Can you work these out from the model? Positions are in its coordinate system, mm. Face numbers are marked on the shaded views. Round coordinates to 2 decimals unless told otherwise and drop trailing zeros. Write each loop counter-clockwise with the first axis right and the second up, starting at its lowest first coordinate (ties: lowest second). Pieces come first, ordered by that corner, then holes. Notation, with made-up numbers: M 64,50.5 L 93,50.5 A16 cw 93,60.5 Z; hole C -27,69.25 d11. An arc over 180 degrees is marked long. Answer as a JSON object with one key per item and string values. Group by question number.
1) Suppose I cut it at A-A, the plane y = 0. Write out the boundary of the cut face in (x, z).
2) If we mould it in two halves opening along Y, with no side actions, what happens to the marked faces 1, 2 and 3? For each: +Y half, -Y half, draft (parallel to the pull), parting line (faces both ways), or undercut.
3) Please list where these lines run through material, in increasing order: L1, parallel to Z at x = 14, y = 0; L2, parallel to Z at x = -17, y = 4.5; L3, parallel to Y at x = -6.5, z = 1. Write a range as [from, to].
4) Suppose I cut it at C-C, the plane x = -7. Write out the boundary of the cut face in (y, z).
5) I'm going to push flat-ended pins straight in: pin 1 Ø2 at (x, z) = (1.5, 4) entering from -Y; pin 2 Ø6 at (y, z) = (-1, 0) entering from -X; pin 3 Ø2 at (x, z) = (19, 2) entering from +Y; pin 4 Ø3 at (x, y) = (0, 4) entering from -Z. Where does each tip first touch, or does it pass through?
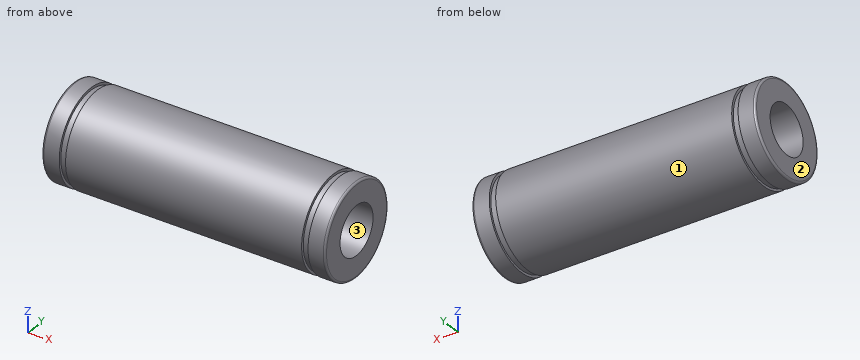
Autodesk Inventor part; units mm, degrees
ref_plane "to_housing_XY" through (0, 0, 0) normal (-1, 0, 0) x (0, 0, -1)
ref_plane "to_housing_YZ" through (0, 0, 0) normal (0, 0, -1) x (0, -1, 0)
ref_plane "to_housing_ZX" through (0, 0, 0) normal (0, -1, 0) x (-1, 0, 0)
sketch "Sketch_1" plane through (0, 0, 0) normal (0, 0, 1) x (1, 0, 0)
  line L0 (28.85, 0) -> (-28.85, 0)
  line L1 (-28.85, 0) -> (-28.85, 9.1)
  arc A0 (-28.45, 9.5) -> (-28.85, 9.1) centre (-28.45, 9.1) ccw
  line L2 (-28.45, 9.5) -> (-25.35, 9.5)
  line L3 (-25.35, 9.5) -> (-25.35, 9)
  line L4 (-25.35, 9) -> (-24.05, 9)
  line L5 (-24.05, 9) -> (-24.05, 9.5)
  line L6 (-24.05, 9.5) -> (24.05, 9.5)
  line L7 (24.05, 9.5) -> (24.05, 9)
  line L8 (24.05, 9) -> (25.35, 9)
  line L9 (25.35, 9) -> (25.35, 9.5)
  line L10 (25.35, 9.5) -> (28.45, 9.5)
  arc A1 (28.85, 9.1) -> (28.45, 9.5) centre (28.45, 9.1) ccw
  line L11 (28.85, 9.1) -> (28.85, 0)
  line L12 (28.85, 0) -> (-28.85, 0)
revolve "Revolution1" add sketch "Sketch_1" angle 360 about axis through (28.85, 0, 0) along (1, 0, 0)
sketch "Sketch2" plane through (28.85, 0, 0) normal (1, 0, 0) x (0, 0, -1)
  point P0 (0, 0)
hole "Hole1" at (28.85, 0, 0) direction (-1, 0, 0) diameter 10 depth 57.7
ref_plane "to_housing_XY" through (0, 0, 0) normal (-1, 0, 0) x (0, 0, -1)
ref_plane "to_housing_YZ" through (0, 0, 0) normal (0, 0, -1) x (0, -1, 0)
ref_plane "to_housing_ZX" through (0, 0, 0) normal (0, -1, 0) x (-1, 0, 0)
properties part number "BUSHING_REFERENCE_DATA_FOR_LHSSW10"
Results:
{
 "1": {"outline": "M -28.85,-9.1 A0.4 ccw -28.45,-9.5 L -25.35,-9.5 L -25.35,-9 L -24.05,-9 L -24.05,-9.5 L 24.05,-9.5 L 24.05,-9 L 25.35,-9 L 25.35,-9.5 L 28.45,-9.5 A0.4 ccw 28.85,-9.1 L 28.85,-5 L -28.85,-5 Z; M -28.85,5 L 28.85,5 L 28.85,9.1 A0.4 ccw 28.45,9.5 L 25.35,9.5 L 25.35,9 L 24.05,9 L 24.05,9.5 L -24.05,9.5 L -24.05,9 L -25.35,9 L -25.35,9.5 L -28.45,9.5 A0.4 ccw -28.85,9.1 Z"},
 "2": {"face 1": "parting line", "face 2": "draft", "face 3": "undercut"},
 "3": {"L1": "[-9.5, -5], [5, 9.5]", "L2": "[-8.37, -2.18], [2.18, 8.37]", "L3": "[-9.45, -4.9], [4.9, 9.45]"},
 "4": {"outline": "C 0,0 d19; hole C 0,0 d10"},
 "5": {"pin 1": "y = -9.01", "pin 2": "through", "pin 3": "y = 9.45", "pin 4": "z = -9.17"}
}
